Can you work these out from the model? Positions are in its coordinate system, mm. A direction names the side the tool comes from. Round coordinates to 2 decimals unless told otherwise and drop trailing zeros. Loops run counter-clockwise (first coordinate to the right, second up) from the corner with the lowest first, then second, coordinate; pieces in that order, holes last.
(1) I want a section at C-C on z = 42. Write out the boundary of the cut face in (x, y).
(2) Will these pins go through, and if not, where does the flat tip stop? pin 1 Ø1 at (x, z) = (47.5, 53) entering from -Y; pin 2 Ø7 at (y, z) = (104.5, 27.5) entering from +X; pin 3 Ø6 at (y, z) = (53.5, 16) entering from -X.
(3) I want a section at D-D on y = 88. Write out the boundary of the cut face in (x, z).
(4) If I drill on line 1 along Z through (x, y) = (25, 98); line 2 along X through (y, z) = (115.5, 25); line 3 along Z through (x, y) = (10.5, 77), over which ranges is the centre line in solid material (lowest first)?
(5) Thinking about a two-plate mould opening in Y: for faces 6 (the face through (9.31, 60.73, 35.43)), 7 (the face through (14, 51.671, 36)), 8 (the face through (48, 126, 36)), which applies, released by +Y, released by -Y, zero draft, split by the parting line, or undercut?
(6) I want a section at B-B on x = 18. Write out the boundary of the cut face in (y, z).
(7) I want a section at A-A on y = 111.5. Write out the boundary of the cut face in (x, z), plus the area to 3 significant figures.
(8) Which directions (+Z, -Z, +X, -X, +Y, -Y) give clear straight access to the entire face, cutting with the end or side of a thin tool? Please do faces 1 (the face through (32, 97, 59)), 2 (the face through (47, 97, 31)), 3 (the face through (32, 35, 36)), 4 (the face through (16.156, 92.129, 35.57)), 5 (the face through (19, 109, 36)).
from build123d import *

# Parameters (mm, degrees)
CONE002_ROLL_ANGLE   = 90
BOX005_W             = 26
BOX005_H             = 50
BOX005_DEPTH         = 40
POCKET_DEPTH         = 40.001
BOX001_W             = 32
BOX001_H             = 17
BOX001_DEPTH         = 46
BOX002_W             = 26
BOX002_H             = 12
BOX002_DEPTH         = 10
BOX003_W             = 26
BOX003_H             = 26
BOX003_DEPTH         = 46
BOX004_W             = 22
BOX004_H             = 36
BOX004_DEPTH         = 35
CYLINDER_R           = 17.5
CYLINDER_DEPTH       = 18
CYLINDER_PITCH_ANGLE = 90
SKETCH001_R          = 1.5
PAD_DEPTH            = 4.5
PAD_DEPTH_BACK       = 5.5
BOX_W                = 36
BOX_H                = 10
BOX_DEPTH            = 50


with BuildPart() as obj1:
    # Cone002 → Cone002 (revolve)
    with BuildSketch(Plane.XZ):
        Polygon((0, 0), (3.9, 0), (4.2, 11), (0, 11), align=None)
    revolve(axis=Axis((0, 0, 0), (0, 0, 1)))


with BuildPart() as obj1_1:
    # Cone002 roll: moved
    add(obj1.part.rotate(Axis((0, 0, 0), (1, 0, 0)), CONE002_ROLL_ANGLE))


with BuildPart() as obj1_2:
    # Cone002 placement: moved
    add(obj1_1.part.moved(Location((32, 35, 35.5))))


with BuildPart() as pocket:
    # Box005 → Box005 (new body)
    with BuildSketch(Plane(origin=(19, 81, 16), x_dir=(1, 0, 0), z_dir=(0, 0, 1))):
        with Locations((13, 25)):
            Rectangle(BOX005_W, BOX005_H)
    extrude(amount=BOX005_DEPTH)

    # Sketch → Pocket (cut, through all)
    with BuildSketch(Plane(origin=(19, 81, 16), x_dir=(1, 0, 0), z_dir=(0, 0, -1))):
        Polygon((0, 0), (0, -1), (2, -1), (4, 0), align=None)
    extrude(amount=-POCKET_DEPTH, mode=Mode.SUBTRACT)


with BuildPart() as obj2:
    # Box001 → Box001 (new body)
    with BuildSketch(Plane(origin=(16, 102, 13), x_dir=(1, 0, 0), z_dir=(0, 0, 1))):
        with Locations((16, 8.5)):
            Rectangle(BOX001_W, BOX001_H)
    extrude(amount=BOX001_DEPTH)


with BuildPart() as obj3:
    # Box002 → Box002 (new body)
    with BuildSketch(Plane(origin=(22, 92, 31), x_dir=(1, 0, 0), z_dir=(0, 0, 1))):
        with Locations((13, 6)):
            Rectangle(BOX002_W, BOX002_H)
    extrude(amount=BOX002_DEPTH)


with BuildPart() as obj4:
    # Box003 → Box003 (new body)
    with BuildSketch(Plane(origin=(20, 77, 13), x_dir=(1, 0, 0), z_dir=(0, 0, 1))):
        with Locations((13, 13)):
            Rectangle(BOX003_W, BOX003_H)
    extrude(amount=BOX003_DEPTH)


with BuildPart() as obj5:
    # Box004 → Box004 (new body)
    with BuildSketch(Plane(origin=(22, 44, 18), x_dir=(1, 0, 0), z_dir=(0, 0, 1))):
        with Locations((11, 18)):
            Rectangle(BOX004_W, BOX004_H)
    extrude(amount=BOX004_DEPTH)


with BuildPart() as obj6:
    # Cylinder → Cylinder (new body)
    with BuildSketch(Plane.XY):
        Circle(CYLINDER_R)
    extrude(amount=CYLINDER_DEPTH)


with BuildPart() as obj6_1:
    # Cylinder pitch: moved
    add(obj6.part.rotate(Axis((0, 0, 0), (0, 1, 0)), CYLINDER_PITCH_ANGLE))


with BuildPart() as obj6_2:
    # Cylinder placement: moved
    add(obj6_1.part.moved(Location((24, 43, 35.5))))


with BuildPart() as obj7:
    # Sketch001 → Pad (new body, two sides)
    with BuildSketch(Plane(origin=(22, 44, 36), x_dir=(1, 0, 0), z_dir=(0, 0, 1))) as pad_sk:
        with BuildLine():
            Line((1.5, 7.670836), (-16.920451, 7.670836))
            ThreePointArc((-20.14616, 11.888508), (-19.57535, 8.982708), (-16.920451, 7.670836))
            Line((-20.14616, 11.888508), (-17.171201, 22.851854))
            ThreePointArc((-12.625578, 34.600006), (-15.204729, 28.844459), (-17.171201, 22.851854))
            Line((-12.625578, 34.600006), (-6.240143, 47.065773))
            ThreePointArc((-6.240143, 47.065773), (-5.840064, 48.144871), (-5.704179, 49.287696))
            Line((-5.704179, 49.287696), (-5.704179, 58.874008))
            Line((-5.704179, 58.874008), (1.5, 58.874008))
            Line((1.5, 58.874008), (1.5, 7.670836))
        make_face()
        with Locations((-11.5, 17.644535)):
            Circle(SKETCH001_R, mode=Mode.SUBTRACT)
    extrude(amount=PAD_DEPTH)
    extrude(pad_sk.sketch, amount=-PAD_DEPTH_BACK)


with BuildPart() as kopf:
    # Box → Box (new body)
    with BuildSketch(Plane(origin=(14, 116, 11), x_dir=(1, 0, 0), z_dir=(0, 0, 1))):
        with Locations((18, 5)):
            Rectangle(BOX_W, BOX_H)
    extrude(amount=BOX_DEPTH)

    # Fusion: union obj2, obj3, obj4, obj5, obj6, obj7
    add(obj2.part)
    add(obj3.part)
    add(obj4.part)
    add(obj5.part)
    add(obj6_2.part)
    add(obj7.part)

    # Cut: cut Pocket
    add(pocket.part, mode=Mode.SUBTRACT)

    # Cut003: cut obj1
    add(obj1_2.part, mode=Mode.SUBTRACT)


solid = kopf.part
Filled sheet:
1. outline: (14, 116) - (16, 116) - (16, 102) - (19, 102) - (19, 126) - (14, 126) - close; (20, 77) - (22, 77) - (22, 44) - (24, 44) - (24, 26.75) - (42, 26.75) - (42, 44) - (44, 44) - (44, 77) - (46, 77) - (46, 102) - (48, 102) - (48, 116) - (50, 116) - (50, 126) - (45, 126) - (45, 81) - (23, 81) - (21, 82) - (20, 82) - close
2. pin 1: stops at y = 102
2. pin 2: stops at x = 48
2. pin 3: stops at x = 22
3. outline: (14.19, 30.5) - (19, 30.5) - (19, 40.5) - (14.19, 40.5) - close; (20, 13) - (46, 13) - (46, 59) - (20, 59) - (20, 56) - (45, 56) - (45, 16) - (20, 16) - close
4. line 1: z = 13 to 16, 56 to 59
4. line 2: x = 16 to 19, 45 to 48
4. line 3: z = 30.5 to 40.5
5. face 6: undercut
5. face 7: released by -Y
5. face 8: released by +Y
6. outline: (51.67, 30.5) - (102, 30.5) - (102, 13) - (116, 13) - (116, 11) - (126, 11) - (126, 61) - (116, 61) - (116, 59) - (102, 59) - (102, 40.5) - (51.67, 40.5) - close
7. outline: (16, 13) - (48, 13) - (48, 59) - (16, 59) - close; hole (19, 16) - (45, 16) - (45, 56) - (19, 56) - close
7. area: 432 mm2
8. face 1: +Z, +X, -X, -Y
8. face 2: -Z, +X, -Y
8. face 3: -Y
8. face 4: +Z, -Z, -X
8. face 5: +Y
